Geometry check sheet. Reference: the model listing, model coordinates, mm. Face numbers are marked on the shaded views. A direction names the side the tool comes from. Coordinates: 2 decimals unless noted, no trailing zeros. Write each loop counter-clockwise with the first axis right and the second up, starting at its lowest first coordinate (ties: lowest second). Pieces come first, ordered by that corner, then holes. Notation, with made-up numbers: M 17,32 L 72,32 A32 cw 72,63 Z; hole C 53,58 d3. An arc over 180 degrees is marked long. Put each result on its own line as item: value. Start each with the question number.
1) Set-up check for the marked faces 4, 5, 6, 7 and 8: record each of +Z, -Z, +X, -X, +Y, -Y from which the full face is reachable in a straight line by a thin tool's end or side.
2) Gauge pin test, flat ends, axial feed: pin 1 (3 mm diameter, centred on y = -10.5, z = 29, fed in from +X); pin 2 (12 mm diameter, centred on y = 2, z = 11.5, fed in from +X); pin 3 (7 mm diameter, centred on x = 43, y = 2, fed in from +Z). Record the tip position at first contact, or that the pin passes through.
3) Cross-section at C-C on x = 43. Record the cut outline in (y, z).
4) Cross-section at B-B on y = -10.5. Record the cut outline in (x, z), plus the area to 3 significant figures.
5) Cross-section at A-A on z = 4. Record the cut outline in (x, y), plus the area to 3 significant figures.
6) Cross-section at D-D on z = 13. Record the cut outline in (x, y), plus the area to 3 significant figures.
7) Mould release check, pull along X, two halves, no side actions. Record for the marked faces 1, 2 and 3: released by +X, released by -X, zero draft, split by the parting line, or undercut.
8) Scan lines: line 1 along X through (y, z) = (3.5, 33.5); line 2 along Z through (x, y) = (79, 3). Record each from-to range of solid material in increasing order.
from build123d import *

# Parameters (mm, degrees)
F0_W     = 16
F0_H     = 4.5
F0_W_2   = 6.5
F0_W_3   = 4
F1_DEPTH = 0.4
F2_W     = 6.5
F2_H     = 4.5
F3_DEPTH = 10
F4_DEPTH = 25


with BuildPart() as f1:
    # F0 (on Top) → F1 (new body)
    with BuildSketch(Plane.XY):
        with BuildLine():
            Line((15.75, 4.75), (15.75, 8.25))
            ThreePointArc((15.75, 8.25), (13.5533008589, 13.5533008589), (8.25, 15.75))
            Line((8.25, 15.75), (-8.25, 15.75))
            ThreePointArc((-8.25, 15.75), (-13.5533008589, 13.5533008589), (-15.75, 8.25))
            Line((-15.75, 8.25), (-15.75, -8.25))
            ThreePointArc((-15.75, -8.25), (-13.5533008589, -13.5533008589), (-8.25, -15.75))
            Line((-8.25, -15.75), (8.25, -15.75))
            ThreePointArc((8.25, -15.75), (13.5533008589, -13.5533008589), (15.75, -8.25))
            Line((15.75, -8.25), (15.75, -4.75))
            Line((15.75, -4.75), (27.3219212057, -4.75))
            ThreePointArc((27.3219212057, -4.75), (32.5853423404, -7.9993666334), (37.75, -4.5952078799))
            ThreePointArc((37.75, -4.5952078799), (42.9146576596, -7.9993666334), (48.1780787943, -4.75))
            Line((48.1780787943, -4.75), (63.9480829801, -4.75))
            ThreePointArc((63.9480829801, -4.75), (69.6474451199, -16.1274567319), (77.3637435709, -6.0087617221))
            Line((77.3637435709, -6.0087617221), (81.5596501878, 1.2587617221))
            ThreePointArc((81.5596501878, 1.2587617221), (83.4749132345, 15.4773568118), (73.9480829801, 4.75))
            Line((73.9480829801, 4.75), (48.1780787943, 4.75))
            ThreePointArc((48.1780787943, 4.75), (42.9146576596, 7.9993666334), (37.75, 4.5952078799))
            ThreePointArc((37.75, 4.5952078799), (32.5853423404, 7.9993666334), (27.3219212057, 4.75))
            Line((27.3219212057, 4.75), (15.75, 4.75))
        make_face()
        with BuildLine():
            ThreePointArc((-13.25, 8.25), (-11.7855339059, 11.7855339059), (-8.25, 13.25))
            Line((-8.25, 13.25), (-4.5, 13.25))
            Line((-4.5, 13.25), (4.5, 13.25))
            Line((4.5, 13.25), (8.25, 13.25))
            ThreePointArc((8.25, 13.25), (11.7855339059, 11.7855339059), (13.25, 8.25))
            Line((13.25, 8.25), (13.25, 4.5))
            Line((13.25, 4.5), (13.25, 2.25))
            Line((13.25, 2.25), (29.25, 2.25))
            ThreePointArc((29.25, 2.25), (32.5, 5.5), (35.75, 2.25))
            Line((35.75, 2.25), (39.75, 2.25))
            ThreePointArc((39.75, 2.25), (43, 5.5), (46.25, 2.25))
            Line((46.25, 2.25), (74.0490381057, 2.25))
            Line((74.0490381057, 2.25), (76.1669476654, 5.9183269633))
            ThreePointArc((76.1669476654, 5.9183269633), (82.8480762114, 12.9903810568), (80.0640619824, 3.6683269633))
            Line((80.0640619824, 3.6683269633), (74.5292047573, -5.9183269633))
            ThreePointArc((74.5292047573, -5.9183269633), (67.8480762114, -12.9903810568), (70.6320904403, -3.6683269633))
            Line((70.6320904403, -3.6683269633), (71.4509618943, -2.25))
            Line((71.4509618943, -2.25), (46.25, -2.25))
            ThreePointArc((46.25, -2.25), (43, -5.5), (39.75, -2.25))
            Line((39.75, -2.25), (35.75, -2.25))
            ThreePointArc((35.75, -2.25), (32.5, -5.5), (29.25, -2.25))
            Line((29.25, -2.25), (13.25, -2.25))
            Line((13.25, -2.25), (13.25, -4.5))
            Line((13.25, -4.5), (13.25, -8.25))
            ThreePointArc((13.25, -8.25), (11.7855339059, -11.7855339059), (8.25, -13.25))
            Line((8.25, -13.25), (4.5, -13.25))
            Line((4.5, -13.25), (-4.5, -13.25))
            Line((-4.5, -13.25), (-8.25, -13.25))
            ThreePointArc((-8.25, -13.25), (-11.7855339059, -11.7855339059), (-13.25, -8.25))
            Line((-13.25, -8.25), (-13.25, -4.5))
            Line((-13.25, -4.5), (-13.25, 4.5))
            Line((-13.25, 4.5), (-13.25, 8.25))
        make_face(mode=Mode.SUBTRACT)
        Polygon((74.0490381057, 2.25), (46.25, 2.25), (46.25, -2.25), (71.4509618943, -2.25), align=None)
        Polygon((4.5, -4.5), (0, -4.5), (-4.5, -4.5), (-4.5, -13.25), (4.5, -13.25), align=None)
        Polygon((-4.5, 0), (-4.5, 4.5), (-13.25, 4.5), (-13.25, -4.5), (-4.5, -4.5), align=None)
        Polygon((4.5, 13.25), (-4.5, 13.25), (-4.5, 4.5), (0, 4.5), (4.5, 4.5), align=None)
        Polygon((13.25, 4.5), (4.5, 4.5), (4.5, 0), (4.5, -4.5), (13.25, -4.5), (13.25, -2.25), (13.25, 2.25), align=None)
        with BuildLine():
            ThreePointArc((80.0640619824, 3.6683269633), (82.8480762114, 12.9903810568), (76.1669476654, 5.9183269633))
            ThreePointArc((76.1669476654, 5.9183269633), (77.8480762114, 4.3301270189), (80.0640619824, 3.6683269633))
        make_face()
        with BuildLine():
            ThreePointArc((74.5292047573, -5.9183269633), (72.8480762114, -4.3301270189), (70.6320904403, -3.6683269633))
            ThreePointArc((70.6320904403, -3.6683269633), (67.8480762114, -12.9903810568), (74.5292047573, -5.9183269633))
        make_face()
        with Locations((21.25, 0)):
            Rectangle(F0_W, F0_H)
        with BuildLine():
            Line((-4.5, -4.5), (-13.25, -4.5))
            Line((-13.25, -4.5), (-13.25, -8.25))
            ThreePointArc((-13.25, -8.25), (-11.7855339059, -11.7855339059), (-8.25, -13.25))
            Line((-8.25, -13.25), (-4.5, -13.25))
            Line((-4.5, -13.25), (-4.5, -4.5))
        make_face()
        with BuildLine():
            Line((8.25, 13.25), (4.5, 13.25))
            Line((4.5, 13.25), (4.5, 4.5))
            Line((4.5, 4.5), (13.25, 4.5))
            Line((13.25, 4.5), (13.25, 8.25))
            ThreePointArc((13.25, 8.25), (11.7855339059, 11.7855339059), (8.25, 13.25))
        make_face()
        with BuildLine():
            Line((13.25, -4.5), (4.5, -4.5))
            Line((4.5, -4.5), (4.5, -13.25))
            Line((4.5, -13.25), (8.25, -13.25))
            ThreePointArc((8.25, -13.25), (11.7855339059, -11.7855339059), (13.25, -8.25))
            Line((13.25, -8.25), (13.25, -4.5))
        make_face()
        with BuildLine():
            Line((-4.5, 13.25), (-8.25, 13.25))
            ThreePointArc((-8.25, 13.25), (-11.7855339059, 11.7855339059), (-13.25, 8.25))
            Line((-13.25, 8.25), (-13.25, 4.5))
            Line((-13.25, 4.5), (-4.5, 4.5))
            Line((-4.5, 4.5), (-4.5, 13.25))
        make_face()
        with BuildLine():
            ThreePointArc((0, 4.5), (-3.1819805153, 3.1819805153), (-4.5, 0))
            ThreePointArc((-4.5, 0), (-3.1819805153, -3.1819805153), (0, -4.5))
            ThreePointArc((0, -4.5), (3.1819805153, -3.1819805153), (4.5, 0))
            ThreePointArc((4.5, 0), (3.1819805153, 3.1819805153), (0, 4.5))
        make_face()
        with BuildLine():
            Line((76.1669476654, 5.9183269633), (74.0490381057, 2.25))
            Line((74.0490381057, 2.25), (71.4509618943, -2.25))
            Line((71.4509618943, -2.25), (70.6320904403, -3.6683269633))
            ThreePointArc((70.6320904403, -3.6683269633), (72.8480762114, -4.3301270189), (74.5292047573, -5.9183269633))
            Line((74.5292047573, -5.9183269633), (80.0640619824, 3.6683269633))
            ThreePointArc((80.0640619824, 3.6683269633), (77.8480762114, 4.3301270189), (76.1669476654, 5.9183269633))
        make_face()
        with Locations((43, 0)):
            Rectangle(F0_W_2, F0_H)
        with Locations((32.5, 0)):
            Rectangle(F0_W_2, F0_H)
        with Locations((37.75, 0)):
            Rectangle(F0_W_3, F0_H)
        with BuildLine():
            Line((46.25, -2.25), (39.75, -2.25))
            ThreePointArc((39.75, -2.25), (43, -5.5), (46.25, -2.25))
        make_face()
        with BuildLine():
            ThreePointArc((35.75, 2.25), (32.5, 5.5), (29.25, 2.25))
            Line((29.25, 2.25), (35.75, 2.25))
        make_face()
        with BuildLine():
            Line((35.75, -2.25), (29.25, -2.25))
            ThreePointArc((29.25, -2.25), (32.5, -5.5), (35.75, -2.25))
        make_face()
        with BuildLine():
            ThreePointArc((46.25, 2.25), (43, 5.5), (39.75, 2.25))
            Line((39.75, 2.25), (46.25, 2.25))
        make_face()
        with BuildLine():
            Line((4.5, 0), (4.5, 4.5))
            Line((4.5, 4.5), (0, 4.5))
            ThreePointArc((0, 4.5), (3.1819805153, 3.1819805153), (4.5, 0))
        make_face()
        with BuildLine():
            Line((0, 4.5), (-4.5, 4.5))
            Line((-4.5, 4.5), (-4.5, 0))
            ThreePointArc((-4.5, 0), (-3.1819805153, 3.1819805153), (0, 4.5))
        make_face()
        with BuildLine():
            ThreePointArc((0, -4.5), (-3.1819805153, -3.1819805153), (-4.5, 0))
            Line((-4.5, 0), (-4.5, -4.5))
            Line((-4.5, -4.5), (0, -4.5))
        make_face()
        with BuildLine():
            Line((4.5, -4.5), (4.5, 0))
            ThreePointArc((4.5, 0), (3.1819805153, -3.1819805153), (0, -4.5))
            Line((0, -4.5), (4.5, -4.5))
        make_face()
    extrude(amount=F1_DEPTH)

    # F2 (on face) → F3 (join)
    with BuildSketch(Plane.XY.offset(0.4)):
        with BuildLine():
            Line((-4.5, 13.25), (-8.25, 13.25))
            ThreePointArc((-8.25, 13.25), (-11.7855339059, 11.7855339059), (-13.25, 8.25))
            Line((-13.25, 8.25), (-13.25, 4.5))
            Line((-13.25, 4.5), (-4.5, 4.5))
            Line((-4.5, 4.5), (-4.5, 13.25))
        make_face()
        Polygon((4.5, 13.25), (-4.5, 13.25), (-4.5, 4.5), (0, 4.5), (4.5, 4.5), align=None)
        with BuildLine():
            Line((8.25, 13.25), (4.5, 13.25))
            Line((4.5, 13.25), (4.5, 4.5))
            Line((4.5, 4.5), (13.25, 4.5))
            Line((13.25, 4.5), (13.25, 8.25))
            ThreePointArc((13.25, 8.25), (11.7855339059, 11.7855339059), (8.25, 13.25))
        make_face()
        Polygon((13.25, 4.5), (4.5, 4.5), (4.5, 0), (4.5, -4.5), (13.25, -4.5), (13.25, -2.25), (13.25, 2.25), align=None)
        with BuildLine():
            Line((13.25, -4.5), (4.5, -4.5))
            Line((4.5, -4.5), (4.5, -13.25))
            Line((4.5, -13.25), (8.25, -13.25))
            ThreePointArc((8.25, -13.25), (11.7855339059, -11.7855339059), (13.25, -8.25))
            Line((13.25, -8.25), (13.25, -4.5))
        make_face()
        Polygon((4.5, -4.5), (0, -4.5), (-4.5, -4.5), (-4.5, -13.25), (4.5, -13.25), align=None)
        with BuildLine():
            Line((-4.5, -4.5), (-13.25, -4.5))
            Line((-13.25, -4.5), (-13.25, -8.25))
            ThreePointArc((-13.25, -8.25), (-11.7855339059, -11.7855339059), (-8.25, -13.25))
            Line((-8.25, -13.25), (-4.5, -13.25))
            Line((-4.5, -13.25), (-4.5, -4.5))
        make_face()
        Polygon((-4.5, 0), (-4.5, 4.5), (-13.25, 4.5), (-13.25, -4.5), (-4.5, -4.5), align=None)
        with BuildLine():
            Line((4.5, 0), (4.5, 4.5))
            Line((4.5, 4.5), (0, 4.5))
            ThreePointArc((0, 4.5), (3.1819805153, 3.1819805153), (4.5, 0))
        make_face()
        with BuildLine():
            Line((4.5, -4.5), (4.5, 0))
            ThreePointArc((4.5, 0), (3.1819805153, -3.1819805153), (0, -4.5))
            Line((0, -4.5), (4.5, -4.5))
        make_face()
        with BuildLine():
            ThreePointArc((0, -4.5), (-3.1819805153, -3.1819805153), (-4.5, 0))
            Line((-4.5, 0), (-4.5, -4.5))
            Line((-4.5, -4.5), (0, -4.5))
        make_face()
        with BuildLine():
            Line((0, 4.5), (-4.5, 4.5))
            Line((-4.5, 4.5), (-4.5, 0))
            ThreePointArc((-4.5, 0), (-3.1819805153, 3.1819805153), (0, 4.5))
        make_face()
        with BuildLine():
            ThreePointArc((0, 4.5), (-3.1819805153, 3.1819805153), (-4.5, 0))
            ThreePointArc((-4.5, 0), (-3.1819805153, -3.1819805153), (0, -4.5))
            ThreePointArc((0, -4.5), (3.1819805153, -3.1819805153), (4.5, 0))
            ThreePointArc((4.5, 0), (3.1819805153, 3.1819805153), (0, 4.5))
        make_face()
        with Locations((32.5, 0)):
            Rectangle(F2_W, F2_H)
        with BuildLine():
            ThreePointArc((35.75, 2.25), (32.5, 5.5), (29.25, 2.25))
            Line((29.25, 2.25), (35.75, 2.25))
        make_face()
        with BuildLine():
            Line((35.75, -2.25), (29.25, -2.25))
            ThreePointArc((29.25, -2.25), (32.5, -5.5), (35.75, -2.25))
        make_face()
        with BuildLine():
            Line((46.25, -2.25), (39.75, -2.25))
            ThreePointArc((39.75, -2.25), (43, -5.5), (46.25, -2.25))
        make_face()
        with Locations((43, 0)):
            Rectangle(F2_W, F2_H)
        with BuildLine():
            ThreePointArc((46.25, 2.25), (43, 5.5), (39.75, 2.25))
            Line((39.75, 2.25), (46.25, 2.25))
        make_face()
        with BuildLine():
            ThreePointArc((72.8480762114, -4.3301270189), (71.7788727151, -3.8693437522), (70.6320904403, -3.6683269633))
            ThreePointArc((70.6320904403, -3.6683269633), (67.8480762114, -12.9903810568), (74.5292047573, -5.9183269633))
            ThreePointArc((74.5292047573, -5.9183269633), (73.7817279741, -5.0256927751), (72.8480762114, -4.3301270189))
        make_face()
        with BuildLine():
            ThreePointArc((80.0640619824, 3.6683269633), (82.8480762114, 12.9903810568), (76.1669476654, 5.9183269633))
            ThreePointArc((76.1669476654, 5.9183269633), (76.9144244486, 5.0256927751), (77.8480762114, 4.3301270189))
            ThreePointArc((77.8480762114, 4.3301270189), (78.9172797076, 3.8693437522), (80.0640619824, 3.6683269633))
        make_face()
    extrude(amount=F3_DEPTH)

    # F4 (add): a face of the model
    f4_faces = [f1.faces().sort_by_distance(p)[0] for p in [
        (0, 0, 10.4),
    ]]
    extrude(f4_faces, amount=F4_DEPTH)


solid = f1.part
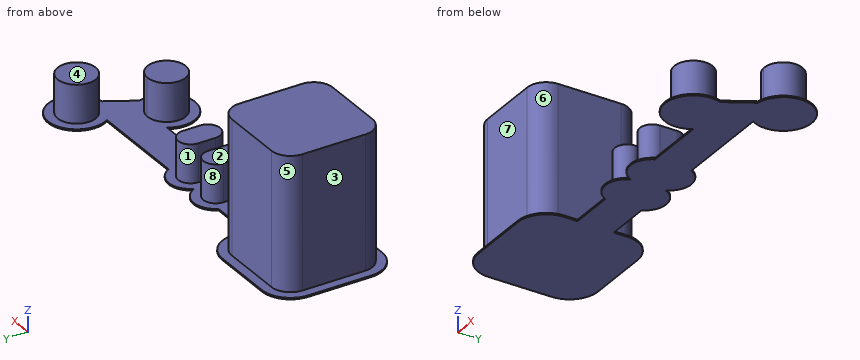
Answer key:
1. face 4: +Z, +X, +Y, -Y
1. face 5: +Z, -X, +Y
1. face 6: +Z, -Y
1. face 7: +Z, -X, -Y
1. face 8: +Z, +Y
2. pin 1: stops at x = 13.19
2. pin 2: stops at x = 85.29
2. pin 3: stops at z = 10.4
3. outline: M -8,0 L 8,0 L 8,0.4 L 5.5,0.4 L 5.5,10.4 L -5.5,10.4 L -5.5,0.4 L -8,0.4 Z
4. outline: M -15.4,0 L 15.4,0 L 15.4,0.4 L 12.72,0.4 L 12.72,35.4 L -12.72,35.4 L -12.72,0.4 L -15.4,0.4 Z; M 63.08,0 L 77.62,0 L 77.62,0.4 L 75,0.4 L 75,10.4 L 65.7,10.4 L 65.7,0.4 L 63.08,0.4 Z
4. area: 1,000 mm²
5. outline: M -13.25,-8.25 A5 ccw -8.25,-13.25 L 8.25,-13.25 A5 ccw 13.25,-8.25 L 13.25,8.25 A5 ccw 8.25,13.25 L -8.25,13.25 A5 ccw -13.25,8.25 Z; M 29.25,-2.25 A3.25 ccw 35.75,-2.25 L 35.75,2.25 A3.25 ccw 29.25,2.25 Z; M 39.75,-2.25 A3.25 ccw 46.25,-2.25 L 46.25,2.25 A3.25 ccw 39.75,2.25 Z; C 70.35,-8.66 d10; C 80.35,8.66 d10
5. area: 963 mm²
6. outline: M -13.25,-8.25 A5 ccw -8.25,-13.25 L 8.25,-13.25 A5 ccw 13.25,-8.25 L 13.25,8.25 A5 ccw 8.25,13.25 L -8.25,13.25 A5 ccw -13.25,8.25 Z
6. area: 681 mm²
7. face 1: undercut
7. face 2: zero draft
7. face 3: released by -X
8. line 1: x = -13.25 to 13.25
8. line 2: z = 0 to 0.4
